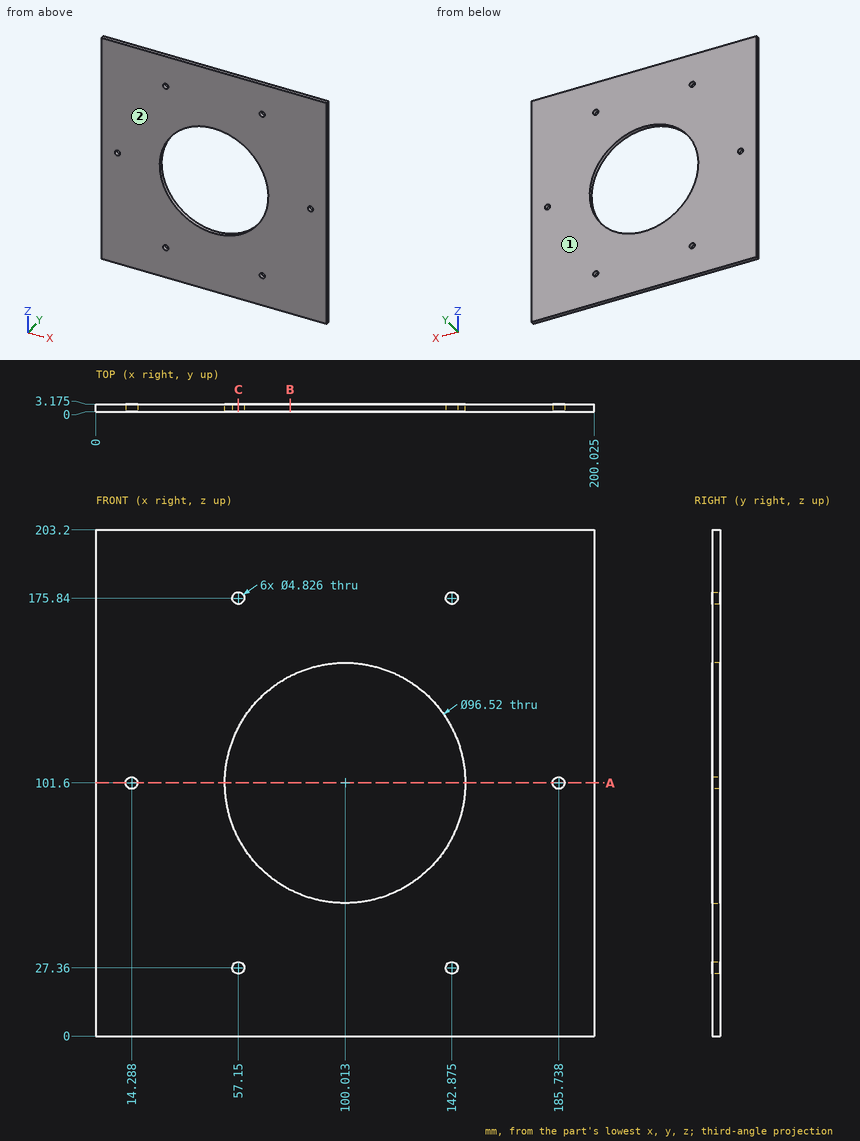
Could you check a few things on this drawing? It's one solid part, dimensions in mm from its lowest x, y, z. Round coordinates to 2 decimals unless told otherwise and drop trailing zeros. Write each loop counter-clockwise with the first axis right and the second up, starting at its lowest first coordinate (ties: lowest second). Pieces come first, ordered by that corner, then holes. Notation, with made-up numbers: (16, -21.5) -> (58, -21.5) arc R29 ccw to (58, -0.5) -> close; hole circle Ø1 at (-24.75, 27). An arc over 180 degrees is marked (long way). One line per question, with ' | ' between items. Start each with the question number.
1) Suppose I cut it at A-A on z = 101.6. Count the separate pieces of the cut face and the enclosed holes in it, then the cut area to 3 significant figures.
2) I need wall thicknesses on line 1 (Z direction, x = 184, y = 2.15) (1 decimal); line 2 (Z direction, x = 60, y = 1.95) (1 decimal); line 3 (X direction, y = 1.7, z = 113) (1 decimal). Which ranges of each line are inside material? Lowest first, please. Write a range as [from, to].
3) Suppose I cut it at B-B on x = 78. Write out the boundary of the cut face in (y, z) (1 decimal).
4) If we mould it in two halves opening along Y, with no side actions, what happens to the marked faces 1 and 2? For each: released by +Y, released by -Y, zero draft, split by the parting line, or undercut.
5) I'm going to push a flat-ended pin straight in: P1, Ø4.5, axis at x = 57.15, z = 27.36, coming from the -Y side. Where does the tip first touch, or does it pass through?
6) Suppose I cut it at C-C on x = 57.15. Write out the boundary of the cut face in (y, z) (1 decimal).
Return value:
1) separate pieces: 4 | enclosed holes: 0 | area: 298 mm2
2) line 1: z = [0, 99.9], [103.3, 203.2] | line 2: z = [0, 74.6], [128.6, 203.2] | line 3: x = [0, 53.1], [146.9, 200]
3) outline: (0, 0) -> (3.2, 0) -> (3.2, 58.7) -> (0, 58.7) -> close; (0, 144.5) -> (3.2, 144.5) -> (3.2, 203.2) -> (0, 203.2) -> close
4) face 1: released by +Y | face 2: released by -Y
5) P1: passes through
6) outline: (0, 0) -> (3.2, 0) -> (3.2, 24.9) -> (0, 24.9) -> close; (0, 29.8) -> (3.2, 29.8) -> (3.2, 79.4) -> (0, 79.4) -> close; (0, 123.8) -> (3.2, 123.8) -> (3.2, 173.4) -> (0, 173.4) -> close; (0, 178.3) -> (3.2, 178.3) -> (3.2, 203.2) -> (0, 203.2) -> close
